Input: part model. Units: mm. Frame: model coordinates. A direction names the side the tool comes from. Coordinates: 2 decimals unless noted, no trailing zeros. Write each loop counter-clockwise with the first axis right and the second up, starting at its lowest first coordinate (ties: lowest second). Pieces come first, ordered by that corner, then holes. Notation, with made-up numbers: M 27.25,53 L 36.25,53 A15 cw 36.25,77 Z; hole C 64,40.25 d5. An arc over 180 degrees is marked long. Use CSV: the item, a comma, the result in double quotes.
Autodesk Inventor part; units mm, degrees
ref_plane "YZ Plane" through (0, 0, 0) normal (1, 0, 0) x (0, 1, 0)
ref_plane "XZ Plane" through (0, 0, 0) normal (0, 1, 0) x (-1, 0, 0)
ref_plane "XY Plane" through (0, 0, 0) normal (0, 0, 1) x (1, 0, 0)
sketch "Skizze_1" plane through (0, 0, 0) normal (0, 0, 1) x (1, 0, 0)
  arc A0 (-4.15, 0.2) -> (-3.95, 0) centre (-3.95, 0.2) ccw
  line L0 (-3.95, 0) -> (4.15, 0)
  arc A1 (4.15, 0) -> (4.35, 0.2) centre (4.15, 0.2) ccw
  line L1 (4.35, 0.2) -> (4.35, 10.1)
  arc A2 (4.35, 10.1) -> (4.15, 10.3) centre (4.15, 10.1) ccw
  line L2 (4.15, 10.3) -> (-3.95, 10.3)
  arc A3 (-3.95, 10.3) -> (-4.15, 10.1) centre (-3.95, 10.1) ccw
  line L3 (-4.15, 10.1) -> (-4.15, 0.2)
extrude "Extrusion1" add sketch "Skizze_1" along normal blind 9.4
sketch "Skizze_2" plane through (0, 0, 0.95) normal (0, 0, 1) x (1, 0, 0)
  line L0 (-2.35, 10.3) -> (-2.35, 2.6)
  line L1 (-2.35, 2.6) -> (2.35, 2.6)
  line L2 (2.35, 2.6) -> (2.35, 10.3)
  line L3 (2.35, 10.3) -> (-2.35, 10.3)
extrude "Extrusion2" cut sketch "Skizze_2" along normal blind 7.5
sketch "Skizze_3" plane through (0, 10.3, 0) normal (0, 1, 0) x (1, 0, 0)
  line L0 (-0.9, -0.95) -> (0.9, -0.95)
  line L1 (0.9, -0.95) -> (0.9, -0.65)
  line L2 (0.9, -0.65) -> (-0.9, -0.65)
  line L3 (-0.9, -0.65) -> (-0.9, -0.95)
extrude "Extrusion3" cut sketch "Skizze_3" against normal blind 7.7
sketch "Skizze_4" plane through (0, 10.3, 0) normal (0, 1, 0) x (1, 0, 0)
  line L0 (-0.9, -8.45) -> (-0.9, -8.75)
  line L1 (-0.9, -8.75) -> (0.9, -8.75)
  line L2 (0.9, -8.75) -> (0.9, -8.45)
  line L3 (0.9, -8.45) -> (-0.9, -8.45)
extrude "Extrusion4" cut sketch "Skizze_4" against normal blind 7.7
sketch "Skizze_5" plane through (0, 10.3, 0) normal (0, 1, 0) x (1, 0, 0)
  line L0 (2.35, -0.95) -> (2.35, -2.9)
  line L1 (2.35, -2.9) -> (3.95, -2.9)
  line L2 (3.95, -2.9) -> (3.95, -0.95)
  line L3 (3.95, -0.95) -> (2.35, -0.95)
extrude "Extrusion5" cut sketch "Skizze_5" against normal blind 6
sketch "Skizze_6" plane through (0, 10.3, 0) normal (0, 1, 0) x (1, 0, 0)
  line L0 (2.35, -6.7) -> (3.95, -6.7)
  line L1 (3.95, -6.7) -> (3.95, -4.75)
  line L2 (3.95, -4.75) -> (2.35, -4.75)
  line L3 (2.35, -4.75) -> (2.35, -6.7)
extrude "Extrusion6" cut sketch "Skizze_6" against normal blind 6
sketch "Skizze_7" plane through (0, 0, 0) normal (0, 1, 0) x (-1, 0, 0)
  line L0 (1.4, 1.7) -> (1.4, 4.5)
  line L1 (1.4, 4.5) -> (-1.4, 4.5)
  line L2 (-1.4, 4.5) -> (-1.4, 1.7)
  line L3 (-1.4, 1.7) -> (1.4, 1.7)
extrude "Extrusion7" add sketch "Skizze_7" along normal blind 3.6
pattern_linear "Rectangular Pattern1" count 2 spacing 3.5 along (0, 0, 1) of "Extrusion7"
sketch "Skizze_9" plane through (0, 0, 0) normal (0, 1, 0) x (-1, 0, 0)
  line L0 (0.5, 2.6) -> (0.5, 3.6)
  line L1 (0.5, 3.6) -> (-0.5, 3.6)
  line L2 (-0.5, 3.6) -> (-0.5, 2.6)
  line L3 (-0.5, 2.6) -> (0.5, 2.6)
extrude "Extrusion8" add sketch "Skizze_9" along normal blind 9.3
pattern_linear "Rectangular Pattern2" count 2 spacing 3.5 along (0, 0, 1) of "Extrusion8"
sketch "Skizze_11" plane through (0, 0, 0) normal (0, 1, 0) x (-1, 0, 0)
  line L0 (0.5, 2.6) -> (0.5, 3.6)
  line L1 (0.5, 3.6) -> (-0.5, 3.6)
  line L2 (-0.5, 3.6) -> (-0.5, 2.6)
  line L3 (-0.5, 2.6) -> (0.5, 2.6)
extrude "Extrusion9" add sketch "Skizze_11" against normal blind 4.5
pattern_linear "Rectangular Pattern3" count 2 spacing 3.5 along (0, 0, 1) of "Extrusion9"
sketch "Skizze_13" plane through (0, 0, 0) normal (0, 1, 0) x (-1, 0, 0)
  line L0 (2.75, 0) -> (2.75, 0.4)
  line L1 (2.75, 0.4) -> (0.9, 0.4)
  line L2 (0.9, 0.4) -> (0.9, 0.65)
  line L3 (0.9, 0.65) -> (-0.9, 0.65)
  line L4 (-0.9, 0.65) -> (-0.9, 0.4)
  line L5 (-0.9, 0.4) -> (-2.75, 0.4)
  line L6 (-2.75, 0.4) -> (-2.75, 0)
  line L7 (-2.75, 0) -> (2.75, 0)
extrude "Extrusion10" cut sketch "Skizze_13" along normal blind 8.3
sketch "Skizze_14" plane through (0, 0, 0) normal (0, 1, 0) x (-1, 0, 0)
  line L0 (2.75, 9.4) -> (-2.75, 9.4)
  line L1 (-2.75, 9.4) -> (-2.75, 9)
  line L2 (-2.75, 9) -> (-0.9, 9)
  line L3 (-0.9, 9) -> (-0.9, 8.75)
  line L4 (-0.9, 8.75) -> (0.9, 8.75)
  line L5 (0.9, 8.75) -> (0.9, 9)
  line L6 (0.9, 9) -> (2.75, 9)
  line L7 (2.75, 9) -> (2.75, 9.4)
extrude "Extrusion11" cut sketch "Skizze_14" along normal blind 8.3
sketch "Skizze_15" plane through (0, 0, 0) normal (0, 1, 0) x (-1, 0, 0)
  line L0 (4.15, 1.8) -> (4.15, 4.4)
  line L1 (4.15, 4.4) -> (2.95, 4.4)
  line L2 (2.95, 4.4) -> (2.95, 1.8)
  line L3 (2.95, 1.8) -> (4.15, 1.8)
extrude "Extrusion12" cut sketch "Skizze_15" along normal blind 9.15
pattern_linear "Rectangular Pattern4" count 2 spacing 3.5 along (0, 0, 1) of "Extrusion12"
sketch "Skizze_17" plane through (0, 0, 0) normal (0, 1, 0) x (-1, 0, 0)
  line L0 (-3.55, 2.55) -> (-3.55, 3.65)
  line L1 (-3.55, 3.65) -> (-4.05, 3.65)
  line L2 (-4.05, 3.65) -> (-4.05, 4.4)
  line L3 (-4.05, 4.4) -> (-4.35, 4.4)
  line L4 (-4.35, 4.4) -> (-4.35, 1.8)
  line L5 (-4.35, 1.8) -> (-4.05, 1.8)
  line L6 (-4.05, 1.8) -> (-4.05, 2.55)
  line L7 (-4.05, 2.55) -> (-3.55, 2.55)
extrude "Extrusion13" cut sketch "Skizze_17" along normal blind 3.9
sketch "Skizze_18" plane through (0, 0, 0) normal (0, 1, 0) x (-1, 0, 0)
  line L0 (-3.55, 6.05) -> (-3.55, 7.15)
  line L1 (-3.55, 7.15) -> (-4.05, 7.15)
  line L2 (-4.05, 7.15) -> (-4.05, 7.9)
  line L3 (-4.05, 7.9) -> (-4.35, 7.9)
  line L4 (-4.35, 7.9) -> (-4.35, 5.3)
  line L5 (-4.35, 5.3) -> (-4.05, 5.3)
  line L6 (-4.05, 5.3) -> (-4.05, 6.05)
  line L7 (-4.05, 6.05) -> (-3.55, 6.05)
extrude "Extrusion14" cut sketch "Skizze_18" along normal blind 3.9
sketch "Sketch15" plane through (-0.5, -4.5, 7.1) normal (0, -1, 0) x (1, 0, 0)
  line L0 (1, -1) -> (0, -1)
  line L1 (0, 0) -> (1, 0)
  line L2 (0, -3.5) -> (1, -3.5)
  line L3 (1, -4.5) -> (0, -4.5)
  line L4 (0, -1) -> (1, 0)
  line L5 (0, -4.5) -> (1, -3.5)
  circle A0 centre (0.5, -4) radius 0.127
  circle A1 centre (0.5, -0.5) radius 0.127
  point P0 (0.5, -7.1)
  dimension "d52" = 0.254
extrude "Extrusion15" cut sketch "Sketch15" against normal blind 0.254
properties part number "734-132"
1. Contact query for flat-ended pins moving along their axis: pin 1 Ø0.5 at (x, y) = (0, 7) entering from -Z; pin 2 Ø1.1 at (y, z) = (-2.5, 3.5) entering from -X; pin 3 Ø1.5 at (x, z) = (3, 2) entering from +Y. Output: stop coordinate, or through.
Resolved:
pin 1,"stops at z = 2.6"
pin 2,"stops at x = -0.5"
pin 3,"stops at y = 4.3"
2. Access query for faces 1 (the flat face through (-2, 4, 0.4)), 2 (the flat face through (3, 4.3, 6)), 3 (the flat face through (0, -2, 6.1)), 4 (the flat face through (0.5, -2.2, 6.6)), 5 (the flat face through (-4, 9.15, 3)). Directions: +Z, -Z, +X, -X, +Y, -Y. A direction counts if a zero-diameter tool reaches every point of the face in a straight line with its end or side. Return the directions, or none.
Resolved:
face 1,"-Z, -Y"
face 2,"+Y"
face 3,"+X, -X, -Y"
face 4,"+Z, -Z, +X, -Y"
face 5,"-X, -Y"
3. Section A-A (y = -3). Return loops of the section in (x, z), then the cut area to 3 significant figures.
Resolved:
outline,"M -0.5,2.6 L 0.5,2.6 L 0.5,3.6 L -0.5,3.6 Z; M -0.5,6.1 L 0.5,6.1 L 0.5,7.1 L -0.5,7.1 Z"
area,"2.00 mm^2"
4. Section B-B (x = 1.75). Return loops of the section in (y, z).
Resolved:
outline,"M 0,0.4 L 8.3,0.4 L 8.3,0 L 10.3,0 L 10.3,0.95 L 2.6,0.95 L 2.6,8.45 L 10.3,8.45 L 10.3,9.4 L 8.3,9.4 L 8.3,9 L 0,9 Z"
5. Material intervals for line 1 (X direction, y = 6, z = 3.25); line 2 (Z direction, x = 2.5, y = 7.5); line 3 (X direction, y = 3.5, z = 7.5), sorted ascending. Write a range as [from, to].
Resolved:
line 1,"x = [-2.95, -2.35], [-0.5, 0.5], [2.35, 4.35]"
line 2,"z = [0.4, 0.95], [2.9, 4.75], [6.7, 9]"
line 3,"x = [-2.95, -2.35], [-1.4, 1.4], [2.35, 4.05]"
6. Section C-C (y = 4.5). State how many separate pieces and enclosed holes the cut face has, then the cut area to 3 significant figures.
Resolved:
separate pieces,"4"
enclosed holes,"0"
area,"27.8 mm^2"
7. Mould query, pull axis X, two halves, no side actions, for faces 6 (the flat face through (-1.4, 3, 3)), 7 (the flat face through (0, 9, 0)), 8 (the flat face through (0.5, -2, 3)). Classes: pulls with the +X half, pulls with the -X half, needs draft (parallel to the pull), parting line crosses it, or undercut.
Resolved:
face 6,"undercut"
face 7,"needs draft"
face 8,"pulls with the +X half"
